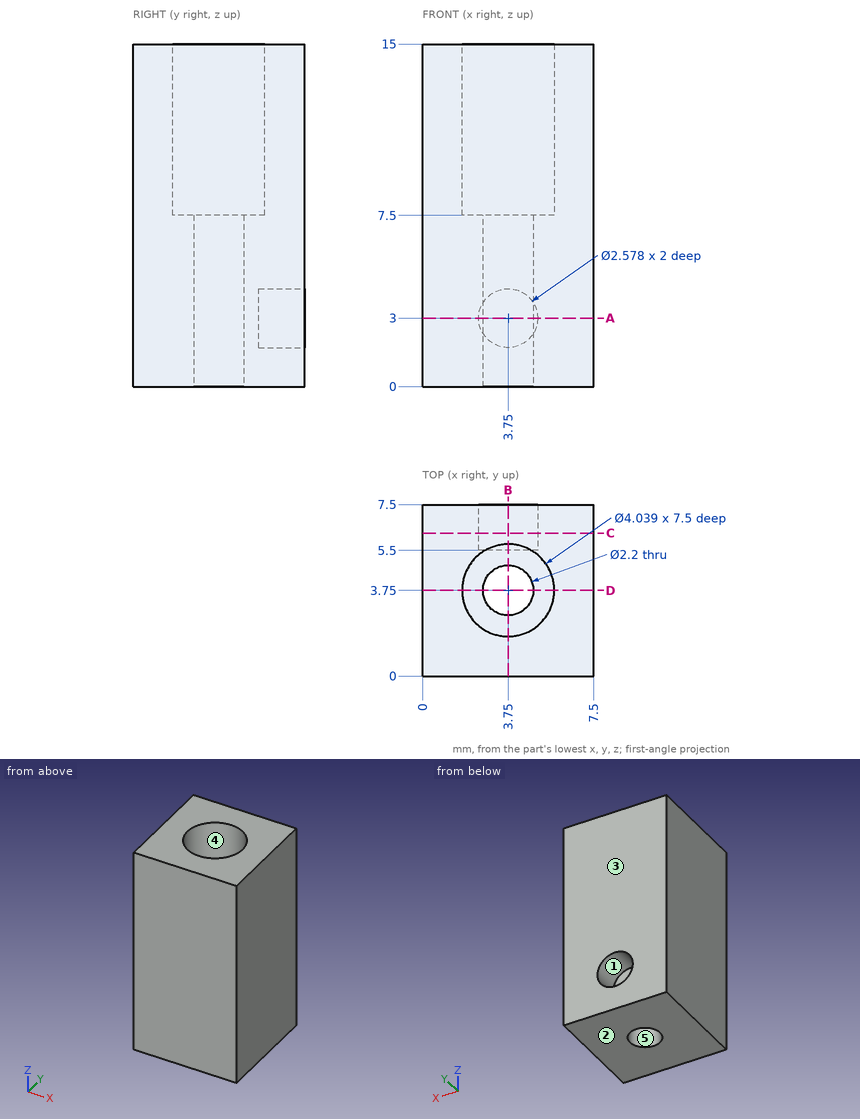
Verification items for this drawing (mm, ordinates from the low corner). A direction names the side the tool comes from. Coordinates: 2 decimals unless noted, no trailing zeros. Order: outer loops, then holes, each group sorted by start corner. A loop starts at its lowest first (then second) coordinate and runs counter-clockwise, first axis right, second up.
Q1. Draft check along Z on the marked faces 1, 2 and 3. Enter one of: released by +Z, released by -Z, zero draft, split by the parting line, or undercut.
Reply:
face 1: undercut
face 2: released by -Z
face 3: zero draft
Q2. Sectioned sample at B-B on x = 3.75. Record the cut outline in (y, z).
Reply:
outline: (0, 0) - (2.65, 0) - (2.65, 7.5) - (1.73, 7.5) - (1.73, 15) - (0, 15) - close; (4.85, 0) - (7.5, 0) - (7.5, 1.71) - (5.5, 1.71) - (5.5, 4.29) - (7.5, 4.29) - (7.5, 15) - (5.77, 15) - (5.77, 7.5) - (4.85, 7.5) - close
Q3. Tool access check on the marked faces 4 and 5. Record the directions out of +Z, -Z, +X, -X, +Y, -Y that give a thin tool (end or side, any length) a straight path to the whole face; none if there is none.
Reply:
face 4: +Z
face 5: +Z, -Z
Q4. Sectioned sample at A-A on z = 3. Record the cut outline in (x, y).
Reply:
outline: (0, 0) - (7.5, 0) - (7.5, 7.5) - (5.04, 7.5) - (5.04, 5.5) - (2.46, 5.5) - (2.46, 7.5) - (0, 7.5) - close; hole circle Ø2.2 at (3.75, 3.75)
Q5. Depth check by flat-ended pin: pin 1 Ø3 at (x, y) = (3.75, 3.75) entering from +Z; pin 2 Ø1.3 at (x, y) = (3.75, 3.75) entering from -Z; pin 3 Ø0.8 at (x, z) = (4, 3) entering from +Y. Enter the tip coordinate at first touch or a pass-through.
Reply:
pin 1: stops at z = 7.5
pin 2: passes through
pin 3: stops at y = 5.5
Q6. Sectioned sample at D-D on y = 3.75. Record the cut outline in (x, z).
Reply:
outline: (0, 0) - (2.65, 0) - (2.65, 7.5) - (1.73, 7.5) - (1.73, 15) - (0, 15) - close; (4.85, 0) - (7.5, 0) - (7.5, 15) - (5.77, 15) - (5.77, 7.5) - (4.85, 7.5) - close
Q7. Sectioned sample at C-C on y = 6.25. Record the cut outline in (x, z).
Reply:
outline: (0, 0) - (7.5, 0) - (7.5, 15) - (0, 15) - close; hole circle Ø2.58 at (3.75, 3)
Q8. Thickness scan on probe 1 along X at (y, z) = (6.85, 3); probe 2 along Y at (x, z) = (3.75, 11.25); probe 3 along Z at (x, y) = (3.75, 6.9). Record the ranges inside material, lowest first.
Reply:
probe 1: x = 0 to 2.46, 5.04 to 7.5
probe 2: y = 0 to 1.73, 5.77 to 7.5
probe 3: z = 0 to 1.71, 4.29 to 15
